Geometry check sheet. Reference: the model listing, model coordinates, mm. A direction names the side the tool comes from. Give positions to 0.01 mm unless a question says otherwise; leave off trailing zeros. Loops run counter-clockwise (first coordinate to the right, second up) from the corner with the lowest first, then second, coordinate; pieces in that order, holes last.
1. Cross-section at C-C, the plane x = 0. Record the cut outline in (y, z), plus the area to 3 significant figures.
2. Go/stop test with a flat-tipped pin: pin 1 Ø2 at (y, z) = (18, 5.5) entering from +X. Record where the tip stops, or that it passes through.
3. Release check for a two-part mould opening along Y. For faces 1 (the flat face through (0, 39.25, 11)), 2 (the cylindrical face through (-0.063, -36.969, 2.406)), 3 (the flat face through (0, 0, 2)) record: +Y half, -Y half, draft (parallel to the pull), parting line (faces both ways), or undercut.
4. Tool access check on faces 4 (the cylindrical face through (2.58, 4.05, 8.49)), 5 (the cylindrical face through (-10.219, 0.438, 2.406)). Record the directions out of +Z, -Z, +X, -X, +Y, -Y that give a thin tool (end or side, any length) a straight path to the whole face; none if there is none.
5. Cross-section at D-D, the plane z = 3.75. Record the cut outline in (x, y), plus the area to 3 significant figures.
6. Cross-section at A-A, the plane z = 9.75. Record the cut outline in (x, y), plus the area to 3 significant figures.
7. Material ranges on L1, parallel to Y at x = 0, z = 11.75; L2, parallel to Y at x = -0.5, z = 3.75; L3, parallel to Z at x = -2.75, y = -31.5, recorded low to high.
8. Cross-section at B-B, the plane y = 0. Record the cut outline in (x, z), plus the area to 3 significant figures.
from build123d import *

# Parameters (mm, degrees)
SKETCH1_W           = 78.5
SKETCH1_H           = 25
BOSS_EXTRUDE1_DEPTH = 15
SKETCH2_R           = 4.8
CUT_EXTRUDE1_DEPTH  = 13
FILLET1_R           = 0.2
FILLET2_R           = 8
FILLET3_R           = 8


with BuildPart() as part:
    # Sketch1 → Boss-Extrude1 (new body)
    with BuildSketch(Plane(origin=(0, 0, 0), x_dir=(0, 1, 0), z_dir=(0, 0, 1))):
        Rectangle(SKETCH1_W, SKETCH1_H)
    extrude(amount=BOSS_EXTRUDE1_DEPTH)

    # Sketch2 → Cut-Extrude1 (cut)
    with BuildSketch(Plane.XY.offset(15)):
        Circle(SKETCH2_R)
    extrude(amount=-CUT_EXTRUDE1_DEPTH, mode=Mode.SUBTRACT)

    # Fillet1
    fillet1_edges = [part.edges().sort_by_distance(p)[0] for p in [
        (-4.8, 0, 15),
    ]]
    fillet(fillet1_edges, radius=FILLET1_R)

    # Fillet2
    fillet2_edges = [part.edges().sort_by_distance(p)[0] for p in [
        (12.5, 39.25, 7.5),
        (12.5, -39.25, 7.5),
        (-12.5, -39.25, 7.5),
        (-12.5, 39.25, 7.5),
    ]]
    fillet(fillet2_edges, radius=FILLET2_R)

    # Fillet3
    fillet3_edges = [part.edges().sort_by_distance(p)[0] for p in [
        (0, -39.25, 0),
        (0, 39.25, 0),
        (12.5, 0, 0),
        (-12.5, 0, 0),
        (-10.156854249, 36.906854249, 0),
        (10.156854249, 36.906854249, 0),
        (10.156854249, -36.906854249, 0),
        (-10.156854249, -36.906854249, 0),
    ]]
    fillet(fillet3_edges, radius=FILLET3_R)


solid = part.part
Result:
1. outline: (-39.25, 8) arc R8 ccw to (-31.25, 0) - (31.25, 0) arc R8 ccw to (39.25, 8) - (39.25, 15) - (5, 15) arc R0.2 ccw to (4.8, 14.8) - (4.8, 2) - (-4.8, 2) - (-4.8, 14.8) arc R0.2 ccw to (-5, 15) - (-39.25, 15) - close
1. area: 1,030 mm2
2. pin 1: stops at x = 12.36
3. face 1: +Y half
3. face 2: -Y half
3. face 3: undercut
4. face 4: +Z
4. face 5: -Z, -X, +Y, -Y
5. outline: (-11.28, -31.25) arc R6.78 ccw to (-4.5, -38.03) - (4.5, -38.03) arc R6.78 ccw to (11.28, -31.25) - (11.28, 31.25) arc R6.78 ccw to (4.5, 38.03) - (-4.5, 38.03) arc R6.78 ccw to (-11.28, 31.25) - close; hole circle Ø9.6 at (0, 0)
5. area: 1,600 mm2
6. outline: (-12.5, -31.25) arc R8 ccw to (-4.5, -39.25) - (4.5, -39.25) arc R8 ccw to (12.5, -31.25) - (12.5, 31.25) arc R8 ccw to (4.5, 39.25) - (-4.5, 39.25) arc R8 ccw to (-12.5, 31.25) - close; hole circle Ø9.6 at (0, 0)
6. area: 1,840 mm2
7. L1: y = -39.25 to -4.8, 4.8 to 39.25
7. L2: y = -38.03 to -4.77, 4.77 to 38.03
7. L3: z = 0 to 15
8. outline: (-12.5, 8) arc R8 ccw to (-4.5, 0) - (4.5, 0) arc R8 ccw to (12.5, 8) - (12.5, 15) - (5, 15) arc R0.2 ccw to (4.8, 14.8) - (4.8, 2) - (-4.8, 2) - (-4.8, 14.8) arc R0.2 ccw to (-5, 15) - (-12.5, 15) - close
8. area: 223 mm2
